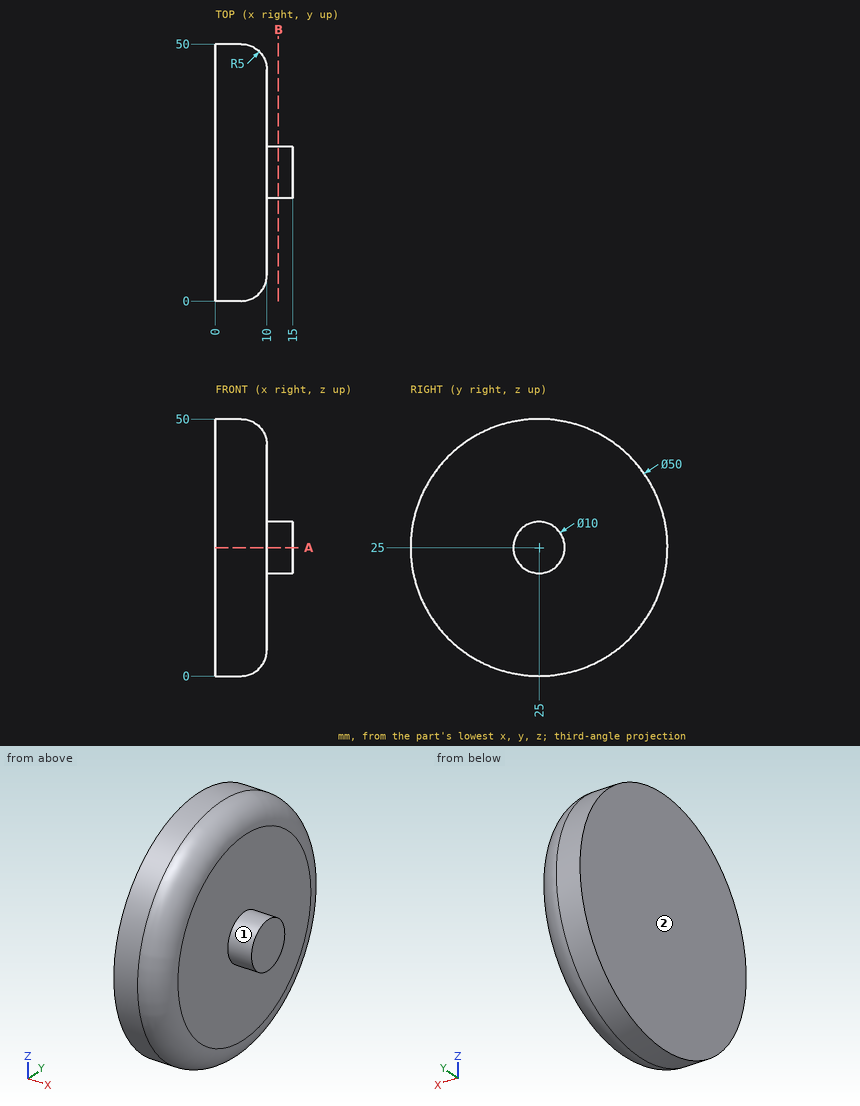
Here's the drawing with two shaded views (mm, measured from the low corner). I have some questions. A direction names the side the tool comes from. Coordinates: 2 decimals unless noted, no trailing zeros. Loops run counter-clockwise (first coordinate to the right, second up) from the corner with the lowest first, then second, coordinate; pieces in that order, holes last. Notation, with made-up numbers: M 9,16 L 68,16 A31 ccw 68,54 Z; hole C 85.5,28.25 d11. An arc over 180 degrees is marked long. Put each result on its own line as item: value. Start each with the question number.
(1) Imagine slicing it at B-B on x = 12.25. List the corners of the cut face in (y, z) for me, and give its area (3 significant figures).
(2) Imagine slicing it at A-A on z = 25. List the corners of the cut face in (x, y) for me, and give its area (3 significant figures).
(3) Will these pins go through, and if not, where does the flat tip stop? pin 1 Ø10 at (y, z) = (21, 7) entering from +X; pin 2 Ø10 at (y, z) = (33.5, 7.5) entering from -X; pin 3 Ø2 at (x, y) = (4.5, 12) entering from -Z; pin 4 Ø1 at (x, z) = (8.5, 16) entering from -Y.
(4) Which directions (+Z, -Z, +X, -X, +Y, -Y) give clear straight access to the entire face, cutting with the end or side of a thin tool? Please do the marked faces 1 and 2.
(5) I need wall thicknesses on probe 1 along X at (y, z) = (18, 33); probe 2 along Y at (x, z) = (4, 22); probe 3 along X at (y, z) = (4, 32). Which ranges of each line are inside material? Lowest first, please.
Worked answers:
1. outline: C 25,25 d10
1. area: 78.5 mm2
2. outline: M 0,0 L 5,0 A5 ccw 10,5 L 10,20 L 15,20 L 15,30 L 10,30 L 10,45 A5 ccw 5,50 L 0,50 Z
2. area: 539 mm2
3. pin 1: stops at x = 10
3. pin 2: stops at x = 0
3. pin 3: stops at z = 3.07
3. pin 4: stops at y = 2.71
4. face 1: +X
4. face 2: +Z, -Z, -X, +Y, -Y
5. probe 1: x = 0 to 10
5. probe 2: y = 0.18 to 49.82
5. probe 3: x = 0 to 9.52
